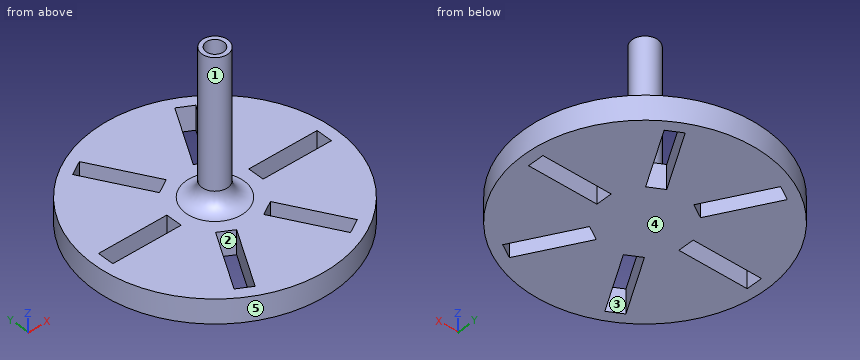
Solid Edge part; units mm, degrees
sketch "Sketch1" plane through (0, 0, 0) normal (0, 0, 1) x (1, 0, 0)
  circle A0 centre (0, 0) radius 15
extrude "Protrusion1" add sketch "Sketch1" along normal blind 3
sketch "Sketch2" plane through (0, 0, 3) normal (0, 0, 1) x (0, 1, 0)
  circle A0 centre (0, 0) radius 1.6
  circle A1 centre (0, 0) radius 1.1
extrude "ExtrudedProtrusion_2" add sketch "Sketch2" along normal blind 18
fillet "Round_1" radius 2 1 edges at (0, -1.6, 3)
sketch "Sketch3" plane through (0, 0, 3) normal (0, 0, 1) x (0, 1, 0)
  line L0 (1, -13.5985) -> (1, -5.0985)
  line L1 (1, -5.0985) -> (-1, -5.0985)
  line L2 (-1, -5.0985) -> (-1, -13.5985)
  line L3 (-1, -13.5985) -> (1, -13.5985)
extrude "Cutout1" cut sketch "Sketch3" against normal up to next
pattern_circular "Pattern1" count 6 over 360 about axis through (0, 0, 3) along (0, 0, 1) of "Cutout1"
Verification items for the finished model (mm, model axes). Face numbers are marked on the shaded views. A direction names the side the tool comes from. Round coordinates to 2 decimals unless told otherwise and drop trailing zeros. Write each loop counter-clockwise with the first axis right and the second up, starting at its lowest first coordinate (ties: lowest second). Pieces come first, ordered by that corner, then holes. Notation, with made-up numbers: (17.5, 68) -> (32.5, 68) arc R26 cw to (32.5, 95) -> close; hole circle Ø1 at (39.5, -23). An arc over 180 degrees is marked (long way). Write each question's results on one line, items separated by ' | '. Start each with the question number.
1. Draft check along Y on the marked faces 3, 4 and 5. Enter one of: +Y half, -Y half, draft (parallel to the pull), parting line (faces both ways), or undercut.
2. Cross-section at B-B (x = 7). Enter the section's corners in (y, z), then the cut area to 3 significant figures.
3. Cross-section at D-D (x = 11.5). Enter the section's corners in (y, z), then the cut area to 3 significant figures.
4. Cross-section at C-C (z = 11.75). Enter the section's corners in (x, y).
5. Cross-section at A-A (y = 0). Enter the section's corners in (x, z).
6. Set-up check for the marked faces 1 and 2: record each of +Z, -Z, +X, -X, +Y, -Y from which the full face is reachable in a straight line by a thin tool's end or side.
7. Material ranges on probe 1 along Y at (x, z) = (0, 9); probe 2 along X at (y, z) = (10.5, 1), recorded low to high. Write a range as from..to.
8. Depth check by flat-ended pin: P1, Ø3.5, axis at x = -11.5, z = 1, coming from the -Y side; P2, Ø1.5, axis at x = 10.5, z = 2, coming from the +Y side; P3, Ø4, axis at x = 0.5, z = 7.5, coming from the +Y side; P4, Ø8, axis at x = 8, z = 13, coming from the -Y side. Enter the tip coordinate at first touch or a pass-through.
Solutions:
1) face 3: undercut | face 4: draft | face 5: parting line
2) outline: (-13.27, 0) -> (-11.66, 0) -> (-11.66, 3) -> (-13.27, 3) -> close; (-10.12, 0) -> (-1, 0) -> (-1, 3) -> (-10.12, 3) -> close; (1, 0) -> (10.12, 0) -> (10.12, 3) -> (1, 3) -> close; (11.66, 0) -> (13.27, 0) -> (13.27, 3) -> (11.66, 3) -> close | area: 64.4 mm2
3) outline: (-9.63, 0) -> (-1, 0) -> (-1, 3) -> (-9.63, 3) -> close; (1, 0) -> (9.63, 0) -> (9.63, 3) -> (1, 3) -> close | area: 51.8 mm2
4) outline: circle Ø3.2 at (0, 0); hole circle Ø2.2 at (0, 0)
5) outline: (-15, 0) -> (-13.6, 0) -> (-13.6, 3) -> (-15, 3) -> close; (-5.1, 0) -> (5.1, 0) -> (5.1, 3) -> (3.6, 3) arc R2 cw to (1.6, 5) -> (1.6, 21) -> (1.1, 21) -> (1.1, 3) -> (-1.1, 3) -> (-1.1, 21) -> (-1.6, 21) -> (-1.6, 5) arc R2 cw to (-3.6, 3) -> (-5.1, 3) -> close; (13.6, 0) -> (15, 0) -> (15, 3) -> (13.6, 3) -> close
6) face 1: +Z | face 2: +Z, -Z
7) probe 1: y = -1.6..-1.1, 1.1..1.6 | probe 2: x = -10.71..-7.22, -4.91..4.91, 7.22..10.71
8) P1: stops at y = -11.4 | P2: stops at y = 11.4 | P3: stops at y = 1.6 | P4: passes through
